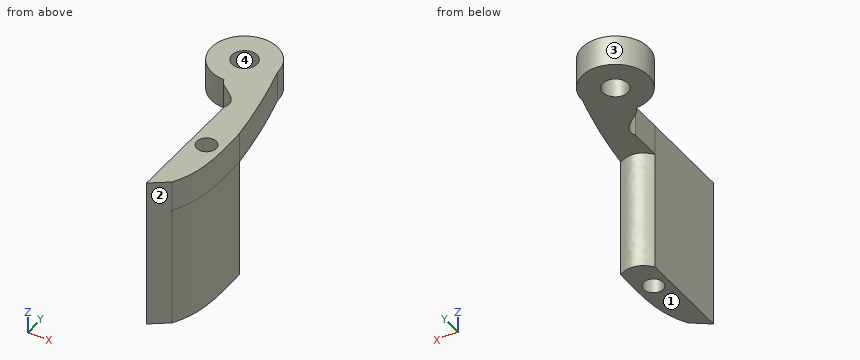
```python
from build123d import *

# Parameters (mm, degrees)
SKETCH1_R           = 2.9
BOSS_EXTRUDE1_DEPTH = 7
BOSS_EXTRUDE2_DEPTH = 27.812432
SKETCH3_R           = 2.25
CUT_EXTRUDE1_DEPTH  = 93.404830354


with BuildPart() as part:
    # Sketch1 → Boss-Extrude1 (new body)
    with BuildSketch(Plane.XY):
        with BuildLine():
            Line((23.684222564, -79.854061858), (27.751665024, -76.911614194))
            add(Edge.make_bspline(
                [(27.751665024, -76.911614194), (30.665612651, -71.996437575), (31.13217948, -67.256532156), (30.668059578, -56.517089881)],
                knots=[0.222415535, 0.222415535, 0.222415535, 0.222415535, 0.766682965, 0.766682965, 0.766682965, 0.766682965], degree=3))
            add(Edge.make_bspline(
                [(30.668059578, -56.517089881), (29.320428981, -45.88374403), (26.453494832, -35.554786486)],
                knots=[0, 0, 0, 1, 1, 1], degree=2))
            ThreePointArc((26.453494832, -35.554786486), (13.359197662, -30.130951008), (18.783033139, -43.225248178))
            add(Edge.make_bspline(
                [(18.783033139, -43.225248178), (19.322772584, -45.817228322), (25.294082339, -46.94058971), (23.583083134, -50.662102957)],
                knots=[0, 0, 0, 0, 1, 1, 1, 1], degree=3))
            Line((23.583083134, -50.662102957), (23.608661583, -58.04483203))
            Line((23.608661583, -58.04483203), (23.684222564, -79.854061858))
        make_face()
        with Locations((18.783033139, -35.554786486)):
            Circle(SKETCH1_R, mode=Mode.SUBTRACT)
    extrude(amount=-BOSS_EXTRUDE1_DEPTH)

    # Sketch2 → Boss-Extrude2 (add)
    with BuildSketch(Plane(origin=(0, 0, -7), x_dir=(-1, 0, 0), z_dir=(0, 0, -1))):
        with BuildLine():
            Line((-27.751665024, -76.911614194), (-23.684222564, -79.854061858))
            Line((-23.684222564, -79.854061858), (-23.608661583, -58.04483203))
            add(Edge.make_bspline(
                [(-23.608661583, -58.04483203), (-26.446360253, -54.336432943), (-30.668059578, -56.51708988)],
                knots=[0, 0, 0, 1, 1, 1], degree=2))
            add(Edge.make_bspline(
                [(-30.668059578, -56.51708988), (-31.132179479, -67.256532155), (-30.665612651, -71.996437575), (-27.751665024, -76.911614194)],
                knots=[0.222415535, 0.222415535, 0.222415535, 0.222415535, 0.766682965, 0.766682965, 0.766682965, 0.766682965], degree=3))
        make_face()
    extrude(amount=BOSS_EXTRUDE2_DEPTH)

    # Sketch3 → Cut-Extrude1 (cut, through all)
    with BuildSketch(Plane.XY):
        with Locations((27.143723241, -63.055671712)):
            Circle(SKETCH3_R)
    extrude(amount=-CUT_EXTRUDE1_DEPTH, mode=Mode.SUBTRACT)


solid = part.part
```
Check sheet for the modelled part. Datum: model origin and axes. Units: mm. Face numbers are marked on the shaded views. Give positions to 0.01 mm unless a question says otherwise; leave off trailing zeros. Order: outer loops, then holes, each group sorted by start corner. A loop starts at its lowest first (then second) coordinate and runs counter-clockwise, first axis right, second up. Notation, with made-up numbers: M 83.5,57 L 113.5,57 A26 ccw 113.5,87 Z; hole C 87,74 d8. An arc over 180 degrees is marked long. Answer in a Markdown table with one row per item.
1) Gauge pin test, flat ends, axial feed: P1, Ø7.5, axis at x = 18.78, y = -35.55, coming from the -Z side; P2, Ø2, axis at x = 26, z = -8.5, coming from the -Y side; P3, Ø6, axis at y = -35.5, z = -7.5, coming from the +X side. Record the tip position at first contact, or that the pin passes through.
Filled sheet:
| item | result |
|---|---|
| P1 | stops at z = -7 |
| P2 | stops at y = -78.9 |
| P3 | stops at x = 27.23 |
2) Cross-section at C-C, the plane z = -2.5. Count the separate pieces of the cut face and the enclosed holes in it, plus the area to 3 significant figures.
Filled sheet:
| item | result |
|---|---|
| separate pieces | 1 |
| enclosed holes | 2 |
| area | 395 mm2 |
3) Cross-section at B-B, the plane x = 18.25. Enter the section's corners in (y, z), plus the area to 3 significant figures.
Filled sheet:
| item | result |
|---|---|
| outline | M -43.21,-7 L -38.41,-7 L -38.41,0 L -43.21,0 Z; M -32.7,-7 L -27.9,-7 L -27.9,0 L -32.7,0 Z |
| area | 67.2 mm2 |
4) Thickness scan on L1, parallel to X at y = -56.5, z = -2; L2, parallel to Y at x = 27, z = -19; L3, parallel to Y at x = 18.75, z = -4. Record the ranges inside material, lowest first. Write a range as [from, to].
Filled sheet:
| item | result |
|---|---|
| L1 | x = [23.6, 30.67] |
| L2 | y = [-77.46, -65.3], [-60.81, -55.77] |
| L3 | y = [-43.23, -38.45], [-32.65, -27.88] |
5) Release check for a two-part mould opening along Y. For the marked faces 1, 2, 3 and 4 record: +Y half, -Y half, draft (parallel to the pull), parting line (faces both ways), or undercut.
Filled sheet:
| item | result |
|---|---|
| face 1 | draft |
| face 2 | -Y half |
| face 3 | parting line |
| face 4 | undercut |
6) Cross-section at D-D, the plane x = 13. Enter the section's corners in (y, z).
Filled sheet:
| item | result |
|---|---|
| outline | M -40.59,-7 L -30.52,-7 L -30.52,0 L -40.59,0 Z |
7) Cross-section at A-A, the plane y = -33.5. Enter the section's corners in (x, z).
Filled sheet:
| item | result |
|---|---|
| outline | M 11.39,-7 L 16.74,-7 L 16.74,0 L 11.39,0 Z; M 20.83,-7 L 26.17,-7 L 26.17,0 L 20.83,0 Z |
